```python
from build123d import *

# Parameters (mm, degrees)
SKETCH1_W           = 10
SKETCH1_H           = 10
BOSS_EXTRUDE1_DEPTH = 15
CUT_EXTRUDE1_DEPTH  = 0.3


with BuildPart() as part:
    # Sketch1 → Boss-Extrude1 (new body)
    with BuildSketch(Plane(origin=(0, 0, 0), x_dir=(1, 0, 0), z_dir=(0, 1, 0))):
        Rectangle(SKETCH1_W, SKETCH1_H)
        with BuildLine():
            Line((-1.658312395, 2.5), (1.658312395, 2.5))
            ThreePointArc((1.658312395, 2.5), (0, -3), (-1.658312395, 2.5))
        make_face(mode=Mode.SUBTRACT)
    extrude(amount=BOSS_EXTRUDE1_DEPTH)

    # Sketch2 → Cut-Extrude1 (cut)
    with BuildSketch(Plane.XY.offset(5)):
        Polygon((0.139535008, 9.754838654), (1.754919623, 6.254838654), (1.413473309, 6.254838654), (0.896045424, 7.376633526), (-0.690593197, 7.376633526), (-1.22274464, 6.254838654), (-1.565593197, 6.254838654), (0.094663213, 9.754838654), align=None)
        Polygon((0.113593501, 9.072647148), (-0.520220601, 7.735607885), (0.730580681, 7.735607885), align=None, mode=Mode.SUBTRACT)
    extrude(amount=-CUT_EXTRUDE1_DEPTH, mode=Mode.SUBTRACT)


solid = part.part
```
Part model, mm, in its own coordinate system. Coordinates: 2 decimals unless noted, no trailing zeros. Write each loop counter-clockwise with the first axis right and the second up, starting at its lowest first coordinate (ties: lowest second). Pieces come first, ordered by that corner, then holes.
Item 1: Mould opens along X. For faces 1 (the face through (5, 7, 0)), 2 (the face through (0, 7, -2.5)), 3 (the face through (2.2, 15, -2.3)) say: released by +X, released by -X, zero draft, split by the parting line, or undercut.
Item 2: Slice it at A-A (z = 2.5). Write the cut outline in (x, y).
Item 3: Probe line 1 (Z direction, x = 0, y = 7.5); line 2 (X direction, y = 6.25, z = 0); line 3 (Z direction, x = 0, y = 12.5). List the from-to ranges inside material, lowest first.
Item 4: Slice it at B-B (x = -2.5). Write the cut outline in (y, z).
Item 5: Slice it at C-C (y = 2.5). Write the cut outline in (x, z).
Results found:
1. face 1: released by +X
1. face 2: undercut
1. face 3: zero draft
2. outline: (-5, 0) - (-1.66, 0) - (-1.66, 15) - (-5, 15) - close; (1.66, 0) - (5, 0) - (5, 15) - (1.66, 15) - close
3. line 1: z = -5 to -2.5, 3 to 4.7
3. line 2: x = -5 to -3, 3 to 5
3. line 3: z = -5 to -2.5, 3 to 5
4. outline: (0, -5) - (15, -5) - (15, -1.66) - (0, -1.66) - close; (0, 1.66) - (15, 1.66) - (15, 5) - (0, 5) - close
5. outline: (-5, -5) - (5, -5) - (5, 5) - (-5, 5) - close; hole (-1.66, -2.5) - (1.66, -2.5) arc R3 ccw (long way) to start
